Verification items for this drawing (mm, ordinates from the low corner). Round coordinates to 2 decimals unless told otherwise and drop trailing zeros. Order: outer loops, then holes, each group sorted by start corner. A loop starts at its lowest first (then second) coordinate and runs counter-clockwise, first axis right, second up. Notation, with made-up numbers: (75, -37.75) -> (117, -37.75) arc R9 cw to (117, -33.75) -> close; hole circle Ø1 at (-38, -3.5). An arc over 180 degrees is marked (long way). Answer in a Markdown table with one row per item. Add a question column.
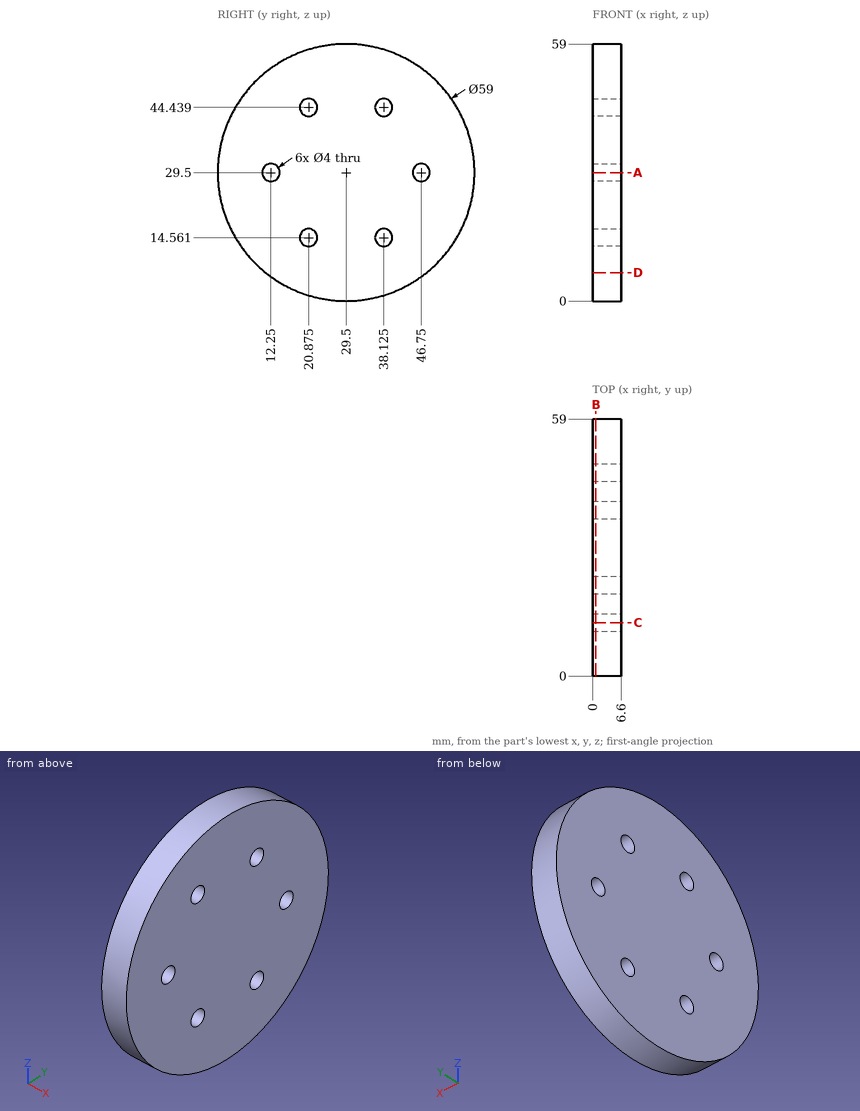
1) Depth check by flat-ended pin: P1, Ø1, axis at x = 4, y = 51, coming from the +Z side; P2, Ø3, axis at y = 38.12, z = 44.44, coming from the -X side; P3, Ø4, axis at y = 24, z = 14.5, coming from the -X side; P4, Ø1.5, axis at x = 2.5, z = 21.5, coming from the +Y side. Enter the tip coordinate at first touch or a pass-through.
2) Thickness scan on L1, parallel to Y at x = 3.25, z = 29.5; L2, parallel to Y at x = 4, z = 28.5; L3, parallel to Z at x = 3.25, y = 20. Record the ranges inside material, lowest first. Write a range as [from, to].
3) Cross-section at B-B, the plane x = 0.75. Record the boundary of the cut face in (y, z) (3 decimals), and give its area (3 significant figures).
4) Cross-section at C-C, the plane y = 12.25. Record the boundary of the cut face in (x, z).
5) Cross-section at D-D, the plane z = 6.5. Record the boundary of the cut face in (x, y), and give its area (3 significant figures).
6) Cross-section at A-A, the plane z = 29.5. Record the boundary of the cut face in (x, y), and give its area (3 significant figures).
Results below:
| question | item | result |
|---|---|---|
| 1 | P1 | z = 50.22 |
| 1 | P2 | through |
| 1 | P3 | x = 0 |
| 1 | P4 | y = 58.1 |
| 2 | L1 | [0, 10.25], [14.25, 44.75], [48.75, 59] |
| 2 | L2 | [0.02, 10.52], [13.98, 45.02], [48.48, 58.98] |
| 2 | L3 | [1.57, 12.76], [16.36, 42.64], [46.24, 57.43] |
| 3 | outline | circle Ø59 at (29.5, 29.5); hole circle Ø4 at (12.25, 29.5); hole circle Ø4 at (20.875, 14.561); hole circle Ø4 at (20.875, 44.439); hole circle Ø4 at (38.125, 14.561); hole circle Ø4 at (38.125, 44.439); hole circle Ø4 at (46.75, 29.5) |
| 3 | area | 2,660 mm² |
| 4 | outline | (0, 5.57) -> (6.6, 5.57) -> (6.6, 27.5) -> (0, 27.5) -> close; (0, 31.5) -> (6.6, 31.5) -> (6.6, 53.43) -> (0, 53.43) -> close |
| 5 | outline | (0, 11.03) -> (6.6, 11.03) -> (6.6, 47.97) -> (0, 47.97) -> close |
| 5 | area | 244 mm² |
| 6 | outline | (0, 0) -> (6.6, 0) -> (6.6, 10.25) -> (0, 10.25) -> close; (0, 14.25) -> (6.6, 14.25) -> (6.6, 44.75) -> (0, 44.75) -> close; (0, 48.75) -> (6.6, 48.75) -> (6.6, 59) -> (0, 59) -> close |
| 6 | area | 337 mm² |
